Model file for the job. Use its own axes, mm. Coordinates: 2 decimals unless noted, no trailing zeros. Loops run counter-clockwise (first coordinate to the right, second up) from the corner with the lowest first, then second, coordinate; pieces in that order, holes last. Notation, with made-up numbers: M 35,86 L 42,86 A24 cw 42,122 Z; hole C 15.5,-18 d9. An arc over 180 degrees is marked long. One line per question, with ' | ' between items. Start each with the question number.
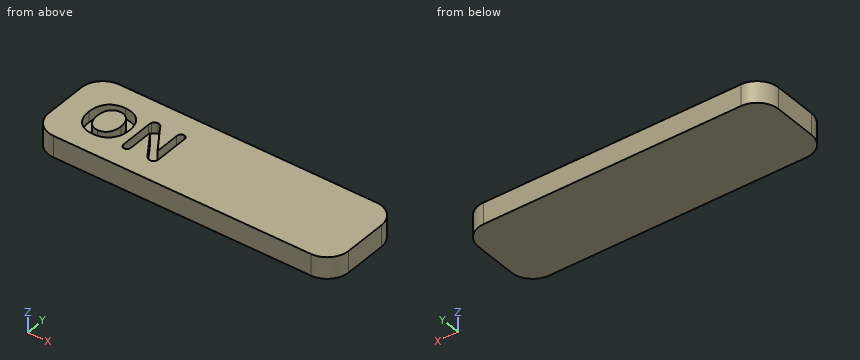
```python
from build123d import *

# Parameters (mm, degrees)
AUFSATZ_LINEAR_AUSTRAGEN1_DEPTH = 1
SCHNITT_LINEAR_AUSTRAGEN1_DEPTH = 0.5


with BuildPart() as part:
    # Skizze1 → Aufsatz-Linear austragen1 (new body)
    with BuildSketch(Plane.XY):
        with BuildLine():
            Line((1, 0), (13, 0))
            ThreePointArc((13, 0), (13.707106781, 0.292893219), (14, 1))
            Line((14, 1), (14, 3))
            ThreePointArc((14, 3), (13.707106781, 3.707106781), (13, 4))
            Line((13, 4), (1, 4))
            ThreePointArc((1, 4), (0.292893219, 3.707106781), (0, 3))
            Line((0, 3), (0, 1))
            ThreePointArc((0, 1), (0.292893219, 0.292893219), (1, 0))
        make_face()
    extrude(amount=AUFSATZ_LINEAR_AUSTRAGEN1_DEPTH)

    # Skizze2 → Schnitt-Linear austragen1 (cut)
    # profile 1 of 2: a face of its own
    with BuildSketch(Plane.XY.offset(1)):
        with BuildLine():
            add(Edge.make_bspline(
                [(2.068359375, 2.975), (2.093112394, 2.974652516), (2.14164836, 2.973971167), (2.213088792, 2.96779492), (2.281989676, 2.95862748), (2.348304365, 2.945431971), (2.411868349, 2.928213747), (2.472693733, 2.90705225), (2.530858895, 2.882017573), (2.586431863, 2.853600887), (2.638802164, 2.821433292), (2.688303235, 2.786256364), (2.73437439, 2.747554036), (2.77712302, 2.705666037), (2.816276383, 2.660478074), (2.852403686, 2.612241049), (2.885226635, 2.56068362), (2.914391718, 2.505816744), (2.940594574, 2.44846024), (2.963340406, 2.388446006), (2.982324979, 2.326028293), (2.998116048, 2.26110371), (3.010084082, 2.193767278), (3.018514176, 2.123861297), (3.024350356, 2.051661497), (3.024781349, 2.002616087), (3.025, 1.977734375)],
                knots=[0, 0, 0, 0, 1.137132438, 2.22970057, 3.292424762, 4.329649132, 5.333981859, 6.315987487, 7.286185149, 8.241436353, 9.181332131, 10.107725602, 11.0292572, 11.943085262, 12.854854597, 13.773819033, 14.709898734, 15.660115542, 16.626635295, 17.605574315, 18.606712189, 19.622473761, 20.67399022, 21.747038223, 22.857027702, 24, 24, 24, 24], degree=3))
            add(Edge.make_bspline(
                [(3.025, 1.977734375), (3.024236943, 1.941248344), (3.022739737, 1.869658489), (3.011382941, 1.76485224), (2.992130943, 1.66508578), (2.965911152, 1.570399581), (2.931448688, 1.481449161), (2.889521373, 1.398351336), (2.839716722, 1.321507209), (2.782571307, 1.250986245), (2.718303636, 1.18718792), (2.646474639, 1.13157047), (2.567529745, 1.084100864), (2.48217021, 1.044116269), (2.38988477, 1.012613038), (2.290860282, 0.991433257), (2.185708374, 0.977018048), (2.11333274, 0.975684634), (2.076171875, 0.975)],
                knots=[0, 0, 0, 0, 1.119700056, 2.196982321, 3.230778928, 4.235358115, 5.208318876, 6.153781848, 7.087131445, 8.013361148, 8.934611457, 9.860297843, 10.794468433, 11.756326826, 12.748403726, 13.780058436, 14.860183413, 16, 16, 16, 16], degree=3))
            add(Edge.make_bspline(
                [(2.076171875, 0.975), (2.03927875, 0.975888232), (1.967053764, 0.977627108), (1.861766869, 0.991561146), (1.762215291, 1.013976035), (1.668967416, 1.04602514), (1.582674595, 1.08683826), (1.502975001, 1.134344554), (1.431414901, 1.190464862), (1.367075118, 1.253597267), (1.309960779, 1.323841341), (1.261404629, 1.401545242), (1.218582067, 1.485017774), (1.184733705, 1.575497068), (1.157803717, 1.671020204), (1.13882396, 1.770875151), (1.127251689, 1.874465923), (1.125758488, 1.944761386), (1.125, 1.98046875)],
                knots=[0, 0, 0, 0, 1.130091603, 2.212359386, 3.247930852, 4.252250901, 5.226719473, 6.16821431, 7.089197795, 8.00610207, 8.925165125, 9.855999165, 10.808795857, 11.79501972, 12.810514548, 13.846493258, 14.906102224, 16, 16, 16, 16], degree=3))
            add(Edge.make_bspline(
                [(1.125, 1.98046875), (1.125688028, 2.016832883), (1.127040936, 2.088337779), (1.139531744, 2.193099625), (1.15925301, 2.293397724), (1.187362441, 2.388727145), (1.223002781, 2.478418194), (1.266262664, 2.561492737), (1.316348518, 2.637693274), (1.373591781, 2.70687478), (1.438083357, 2.768616063), (1.509462446, 2.82261175), (1.587377693, 2.86905948), (1.671832678, 2.907263474), (1.762443164, 2.937927219), (1.859185583, 2.959576748), (1.961878055, 2.97269235), (2.032251673, 2.974217478), (2.068359375, 2.975)],
                knots=[0, 0, 0, 0, 1.125218611, 2.212582392, 3.260701818, 4.286054269, 5.284468473, 6.243521648, 7.180287843, 8.101949555, 9.017004541, 9.937572836, 10.866572707, 11.818894766, 12.801573564, 13.82236102, 14.882684417, 16, 16, 16, 16], degree=3))
        make_face()
        with BuildLine():
            add(Edge.make_bspline(
                [(2.625, 1.98046875), (2.624236115, 2.015277472), (2.622757058, 2.082675226), (2.609648511, 2.180171038), (2.588416712, 2.27060321), (2.563111057, 2.340625009), (2.538811369, 2.392528468), (2.51896586, 2.42865343), (2.497617935, 2.462663361), (2.473388511, 2.493425176), (2.448255174, 2.522406317), (2.421043849, 2.54892338), (2.391707134, 2.572581535), (2.350596581, 2.601296683), (2.295234429, 2.631050621), (2.223753123, 2.656546627), (2.147556711, 2.672258276), (2.09512819, 2.674073293), (2.068359375, 2.675)],
                knots=[0, 0, 0, 0, 1.663767962, 3.22144036, 4.693807908, 6.09809827, 6.772124886, 7.43249818, 8.068074837, 8.689496673, 9.30272399, 9.901527182, 10.503429657, 11.102750509, 12.297797107, 13.495176895, 14.721094103, 16, 16, 16, 16], degree=3))
            add(Edge.make_bspline(
                [(2.068359375, 2.675), (2.04918449, 2.674523021), (2.011287158, 2.673580316), (1.955655243, 2.664627547), (1.902215528, 2.650626376), (1.851216647, 2.631043473), (1.803112784, 2.606035103), (1.758119138, 2.575673263), (1.716778265, 2.540076152), (1.678858763, 2.499387916), (1.64458724, 2.453198562), (1.614182017, 2.401028966), (1.587690016, 2.342878426), (1.565104568, 2.279265806), (1.547241689, 2.210518214), (1.534540277, 2.137356433), (1.526561269, 2.060201883), (1.525528163, 2.007441739), (1.525, 1.98046875)],
                knots=[0, 0, 0, 0, 0.926902171, 1.831933723, 2.71800685, 3.595261319, 4.468550136, 5.334998465, 6.214894287, 7.1017058, 8.020008637, 8.99111482, 10.01694856, 11.106630737, 12.25237115, 13.448355624, 14.695502513, 16, 16, 16, 16], degree=3))
            add(Edge.make_bspline(
                [(1.525, 1.98046875), (1.525529621, 1.953235833), (1.526565779, 1.899956987), (1.534528502, 1.822019496), (1.547312827, 1.74796955), (1.565048146, 1.678113625), (1.58799262, 1.613266121), (1.615536195, 1.554021234), (1.646413772, 1.499956378), (1.682840272, 1.452579062), (1.722186978, 1.410770889), (1.76447307, 1.374356244), (1.809393417, 1.343334803), (1.857378179, 1.318080366), (1.908164293, 1.299131658), (1.961190349, 1.284770984), (2.016800589, 1.276568573), (2.054661701, 1.275527183), (2.073828125, 1.275)],
                knots=[0, 0, 0, 0, 1.300369924, 2.54406124, 3.737115199, 4.88637188, 5.981883645, 7.016846829, 8.003376514, 8.948590554, 9.863559023, 10.741055788, 11.608647785, 12.46534091, 13.323432129, 14.192248925, 15.0848625, 16, 16, 16, 16], degree=3))
            add(Edge.make_bspline(
                [(2.073828125, 1.275), (2.098514049, 1.275826804), (2.147153697, 1.277455889), (2.218375005, 1.292666561), (2.286422084, 1.316581814), (2.340300617, 1.34411813), (2.380907534, 1.371243102), (2.410251531, 1.394127245), (2.437531132, 1.420168305), (2.463533565, 1.448361043), (2.487628227, 1.479320201), (2.510440944, 1.51265316), (2.531503359, 1.54871627), (2.550989754, 1.587307904), (2.568587312, 1.628357856), (2.583936454, 1.67175711), (2.596172475, 1.717696454), (2.606851743, 1.765749251), (2.614975974, 1.816231574), (2.620753103, 1.868901619), (2.624372846, 1.923907557), (2.624787704, 1.961322387), (2.625, 1.98046875)],
                knots=[0, 0, 0, 0, 1.468568495, 2.893578421, 4.316075305, 5.755382189, 6.482330971, 7.222315454, 7.968369796, 8.725783183, 9.504530818, 10.302500265, 11.129737207, 11.9897977, 12.875655565, 13.787998707, 14.728608307, 15.705132475, 16.718642732, 17.771954593, 18.859838044, 20, 20, 20, 20], degree=3))
        make_face(mode=Mode.SUBTRACT)
    # profile 2 of 2: a face of its own
    with BuildSketch(Plane.XY.offset(1)):
        with BuildLine():
            Line((3.86484375, 2.740234375), (4.625, 1.6))
            Line((4.625, 1.6), (4.625, 2.75078125))
            add(Edge.make_bspline(
                [(4.625, 2.75078125), (4.625586836, 2.768395927), (4.626686005, 2.801389002), (4.635036402, 2.847648409), (4.649668068, 2.886889392), (4.670402191, 2.919114128), (4.696180986, 2.944318069), (4.726619023, 2.962223197), (4.761117632, 2.973196011), (4.785463851, 2.974385321), (4.798046875, 2.975)],
                knots=[0, 0, 0, 0, 1.319117216, 2.470765316, 3.505116792, 4.43580569, 5.318756254, 6.18027265, 7.059497782, 8, 8, 8, 8], degree=3))
            add(Edge.make_bspline(
                [(4.798046875, 2.975), (4.811012753, 2.974373778), (4.836109378, 2.97316167), (4.871600638, 2.962412213), (4.902620124, 2.944321241), (4.928806854, 2.919151114), (4.949918941, 2.886925272), (4.965064382, 2.847732261), (4.973280664, 2.80137765), (4.974401563, 2.768391976), (4.975, 2.75078125)],
                knots=[0, 0, 0, 0, 0.959871134, 1.857917088, 2.719075999, 3.600089629, 4.526699118, 5.554128738, 6.694173474, 8, 8, 8, 8], degree=3))
            Line((4.975, 2.75078125), (4.975, 1.2296875))
            add(Edge.make_bspline(
                [(4.975, 1.2296875), (4.974517449, 1.209721265), (4.973611757, 1.172246954), (4.963962629, 1.119848054), (4.947690056, 1.075246898), (4.924922255, 1.038240953), (4.894956518, 1.009207633), (4.857911429, 0.989251615), (4.814719484, 0.976787702), (4.783815821, 0.975615768), (4.767578125, 0.975)],
                knots=[0, 0, 0, 0, 1.276164049, 2.395212213, 3.391561633, 4.297456637, 5.151673506, 6.027862746, 6.963780962, 8, 8, 8, 8], degree=3))
            add(Edge.make_bspline(
                [(4.767578125, 0.975), (4.751115635, 0.975772416), (4.719363897, 0.977262199), (4.673622221, 0.988138948), (4.632032835, 1.008430687), (4.594663962, 1.037771284), (4.55968076, 1.073356467), (4.527659202, 1.11463191), (4.497490318, 1.159350157), (4.476842172, 1.189466295), (4.46640625, 1.2046875)],
                knots=[0, 0, 0, 0, 0.990229924, 1.909888509, 2.806876858, 3.75171819, 4.754420985, 5.802993103, 6.889595585, 8, 8, 8, 8], degree=3))
            Line((4.46640625, 1.2046875), (3.725, 2.325))
            Line((3.725, 2.325), (3.725, 1.198046875))
            add(Edge.make_bspline(
                [(3.725, 1.198046875), (3.724414523, 1.180824483), (3.72330548, 1.148200888), (3.714742096, 1.102326501), (3.698988566, 1.0631574), (3.677344387, 1.0309462), (3.650765302, 1.005883739), (3.620379665, 0.987840533), (3.586282235, 0.976836674), (3.562322205, 0.975623773), (3.55, 0.975)],
                knots=[0, 0, 0, 0, 1.293064309, 2.449392962, 3.484384031, 4.441729672, 5.340986808, 6.204611779, 7.076664708, 8, 8, 8, 8], degree=3))
            add(Edge.make_bspline(
                [(3.55, 0.975), (3.537415957, 0.975600427), (3.512903847, 0.976769981), (3.478206619, 0.988073985), (3.447689985, 1.006729195), (3.421040174, 1.031933145), (3.400304093, 1.064751921), (3.385493226, 1.103922858), (3.376597599, 1.149477245), (3.375553408, 1.181988306), (3.375, 1.19921875)],
                knots=[0, 0, 0, 0, 0.938889884, 1.828837584, 2.693878765, 3.596100726, 4.546832571, 5.570326044, 6.712304089, 8, 8, 8, 8], degree=3))
            Line((3.375, 1.19921875), (3.375, 2.69140625))
            add(Edge.make_bspline(
                [(3.375, 2.69140625), (3.37514655, 2.706394453), (3.375423663, 2.734735734), (3.379522399, 2.774642207), (3.385123318, 2.80976372), (3.392066316, 2.830792867), (3.3953125, 2.840625)],
                knots=[0, 0, 0, 0, 1.18793306, 2.246269525, 3.180047019, 4, 4, 4, 4], degree=3))
            add(Edge.make_bspline(
                [(3.3953125, 2.840625), (3.399668454, 2.850192085), (3.408364875, 2.869292239), (3.427434086, 2.894600683), (3.449198834, 2.91818821), (3.475465064, 2.937620764), (3.503805632, 2.954136488), (3.533862342, 2.966343001), (3.565275925, 2.973670728), (3.5865505, 2.974554753), (3.597265625, 2.975)],
                knots=[0, 0, 0, 0, 0.980600708, 1.957714689, 2.948627098, 3.97434472, 5.000279326, 6.011426356, 6.998437519, 8, 8, 8, 8], degree=3))
            add(Edge.make_bspline(
                [(3.597265625, 2.975), (3.613277137, 2.974362991), (3.643301645, 2.973168483), (3.684701728, 2.959340883), (3.719945443, 2.939070857), (3.750422654, 2.911403027), (3.779239652, 2.877209196), (3.805947743, 2.835053519), (3.834869484, 2.788741916), (3.854699923, 2.756650193), (3.86484375, 2.740234375)],
                knots=[0, 0, 0, 0, 1.01695463, 1.906975685, 2.751376853, 3.592506721, 4.517315556, 5.594915983, 6.76973195, 8, 8, 8, 8], degree=3))
        make_face()
    extrude(amount=-SCHNITT_LINEAR_AUSTRAGEN1_DEPTH, mode=Mode.SUBTRACT)


solid = part.part
```
(1) Band-saw the part on C-C on x = 4.25. Write the cut outline in (y, z).
(2) Band-saw the part on B-B on z = 0.3. Write the cut outline in (x, y), then the cut area to 3 significant figures.
(3) Band-saw the part on A-A on z = 0.85. Give the number of separate pieces and of enclosed holes in the cut face, then the cut area to 3 significant figures.
(4) Band-saw the part on D-D on y = 0.55. Write the cut outline in (x, z).
(5) Drill centre lines: line 1 (X direction, y = 2.85, z = 0.7); line 2 (X direction, y = 1.95, z = 0.95) (3 decimals); line 3 (X direction, y = 3.05, z = 0.9). Where is each one in solid material? Low to high. Write a range as [from, to].
Computed values:
1) outline: M 0,0 L 4,0 L 4,1 L 2.16,1 L 2.16,0.5 L 1.53,0.5 L 1.53,1 L 0,1 Z
2) outline: M 0,1 A1 ccw 1,0 L 13,0 A1 ccw 14,1 L 14,3 A1 ccw 13,4 L 1,4 A1 ccw 0,3 Z | area: 55.1 mm^2
3) separate pieces: 2 | enclosed holes: 2 | area: 51.4 mm^2
4) outline: M 0.11,0 L 13.89,0 L 13.89,1 L 0.11,1 Z
5) line 1: [0, 1.56], [2.59, 3.4], [3.8, 4.64], [4.96, 14] | line 2: [0, 1.126], [1.526, 2.625], [3.024, 3.375], [3.725, 3.973], [4.392, 4.625], [4.975, 14] | line 3: [0, 14]
